```python
from build123d import *

# Parameters (mm, degrees)
SKETCH002_W       = 13
SKETCH002_H       = 26
SKETCH002_W_2     = 3
SKETCH002_H_2     = 16
PAD002_DEPTH      = 36
CYLINDER002_R     = 2.5
CYLINDER002_DEPTH = 14
SKETCH003_W       = 26
SKETCH003_H       = 13
PAD003_DEPTH      = 90
SKETCH004_W       = 16
SKETCH004_H       = 16
PAD004_DEPTH      = 8
CYLINDER003_R     = 2
CYLINDER003_DEPTH = 15


with BuildPart() as part:
    # Sketch002 → Pad002 (new body)
    with BuildSketch(Plane.XY):
        with Locations((1, 0)):
            Rectangle(SKETCH002_W, SKETCH002_H)
        with Locations((1, 0)):
            Rectangle(SKETCH002_W_2, SKETCH002_H_2, mode=Mode.SUBTRACT)
    extrude(amount=-PAD002_DEPTH)

    # Cylinder002 → Cylinder002 (cut)
    with BuildSketch(Plane(origin=(-6, 0, -28.5), x_dir=(0, 1, 0), z_dir=(1, 0, 0))):
        Circle(CYLINDER002_R)
    extrude(amount=CYLINDER002_DEPTH, mode=Mode.SUBTRACT)

    # Sketch003 (on Face4 of Cylinder002) → Pad003 (join)
    with BuildSketch(Plane(origin=(-6, 0, -36), x_dir=(0, 1, 0), z_dir=(0, 0, -1))):
        with Locations((0, 7)):
            Rectangle(SKETCH003_W, SKETCH003_H)
    extrude(amount=PAD003_DEPTH)

    # Sketch004 (on Face14 of Pad003) → Pad004 (join)
    with BuildSketch(Plane(origin=(-6, 0, -126), x_dir=(0, 1, 0), z_dir=(0, 0, -1))):
        with Locations((0, 7)):
            Rectangle(SKETCH004_W, SKETCH004_H)
    extrude(amount=PAD004_DEPTH)

    # Cylinder003 → Cylinder003 (cut)
    with BuildSketch(Plane(origin=(1, 0, -134), x_dir=(1, 0, 0), z_dir=(0, 0, 1))):
        Circle(CYLINDER003_R)
    extrude(amount=CYLINDER003_DEPTH, mode=Mode.SUBTRACT)


with BuildPart() as part_1:
    # Body002 placement: moved
    add(part.part.moved(Location((0, 0, -66))))


solid = part_1.part
```
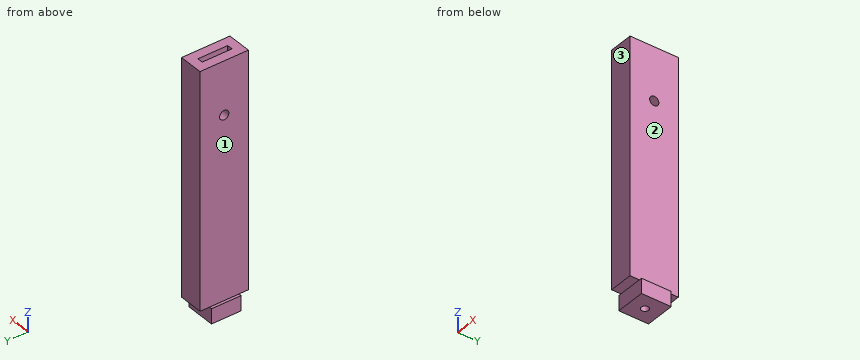
Can you work these out from the model? Positions are in its coordinate system, mm. Face numbers are marked on the shaded views. A direction names the side the tool comes from. Coordinates: 2 decimals unless noted, no trailing zeros. Loops run counter-clockwise (first coordinate to the right, second up) from the corner with the lowest first, then second, coordinate; pieces in that order, holes last. Notation, with made-up numbers: (35.5, 57.25) -> (46.5, 57.25) arc R17 cw to (46.5, 73.25) -> close; hole circle Ø1 at (-18.75, -31.5). An arc over 180 degrees is marked (long way). Put each result on its own line as item: value. Start each with the question number.
Q1. For the marked faces 1, 2 and 3, which set-ups out of +Z, -Z, +X, -X, +Y, -Y let a thin tool reach every point of the face, with its end or its side?
Q2. I want a section at C-C (x = 5.25). Write out the boundary of the cut face in (y, z), plus the area to 3 significant figures.
Q3. I'm going to push flat-ended pins straight in: P1, Ø9, axis at x = 0.5, z = -197, coming from the +Y side; P2, Ø0.8, axis at x = -6, y = -2, coming from the +Z side; P3, Ø0.9, axis at x = 0.5, y = 3, coming from the +Z side. Where does each tip first touch, or does it pass through?
Q4. I want a section at A-A (y = 0). Write out the boundary of the cut face in (x, z), plus the area to 3 significant figures.
Q5. I want a section at D-D (z = -94.5). Write out the boundary of the cut face in (x, y), plus the area to 3 significant figures.
Q6. If I drill on line 1 (X direction, y = -7.25, z = -91); line 2 (Y direction, x = 6.25, z = -94.5); line 3 (X direction, y = -2.75, z = -176), over which ranges is the centre line in solid material (lowest first)? Write a range as [from, to].
Q7. I want a section at B-B (z = -80). Write out the boundary of the cut face in (x, y), plus the area to 3 significant figures.
Taken from the geometry:
1. face 1: +Z, -X, +Y, -Y
1. face 2: +Z, +X, +Y, -Y
1. face 3: +Z, -Z, +X, -X, -Y
2. outline: (-13, -192) -> (-8, -192) -> (-8, -200) -> (8, -200) -> (8, -192) -> (13, -192) -> (13, -66) -> (-13, -66) -> close; hole circle Ø5 at (0, -94.5)
2. area: 3,380 mm2
3. P1: stops at y = 8
3. P2: stops at z = -192
3. P3: stops at z = -102
4. outline: (-7, -200) -> (-1, -200) -> (-1, -185) -> (3, -185) -> (3, -200) -> (9, -200) -> (9, -192) -> (7.5, -192) -> (7.5, -97) -> (2.5, -97) -> (2.5, -102) -> (-0.5, -102) -> (-0.5, -97) -> (-5.5, -97) -> (-5.5, -192) -> (-7, -192) -> close; (-5.5, -92) -> (-0.5, -92) -> (-0.5, -66) -> (-5.5, -66) -> close; (2.5, -92) -> (7.5, -92) -> (7.5, -66) -> (2.5, -66) -> close
4. area: 1,550 mm2
5. outline: (-5.5, -13) -> (7.5, -13) -> (7.5, -2.5) -> (2.5, -2.5) -> (2.5, -8) -> (-0.5, -8) -> (-0.5, -2.5) -> (-5.5, -2.5) -> close; (-5.5, 2.5) -> (-0.5, 2.5) -> (-0.5, 8) -> (2.5, 8) -> (2.5, 2.5) -> (7.5, 2.5) -> (7.5, 13) -> (-5.5, 13) -> close
5. area: 240 mm2
6. line 1: x = [-5.5, -0.5], [2.5, 7.5]
6. line 2: y = [-13, -2.5], [2.5, 13]
6. line 3: x = [-5.5, 7.5]
7. outline: (-5.5, -13) -> (7.5, -13) -> (7.5, 13) -> (-5.5, 13) -> close; hole (-0.5, -8) -> (2.5, -8) -> (2.5, 8) -> (-0.5, 8) -> close
7. area: 290 mm2
